Model file for the job. Use its own axes, mm. Coordinates: 2 decimals unless noted, no trailing zeros. Loops run counter-clockwise (first coordinate to the right, second up) from the corner with the lowest first, then second, coordinate; pieces in that order, holes last. Notation, with made-up numbers: (-26.75, 56.5) -> (-0.75, 56.5) arc R21 ccw to (-0.75, 76.5) -> close; hole circle Ø7 at (78.25, 67). An arc over 180 degrees is marked (long way). Use one line per item in the form item = value.
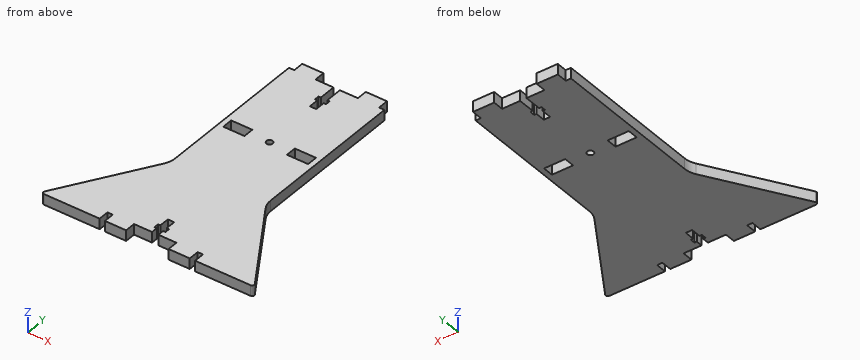
```python
from build123d import *

# Parameters (mm, degrees)
BOSS_EXTRUDE1_DEPTH = 5
SKETCH2_R           = 1.5
SKETCH2_W           = 10
SKETCH2_H           = 5
CUT_EXTRUDE1_DEPTH  = 10
FILLET1_R           = 10
FILLET2_R           = 1


with BuildPart() as part:
    # Sketch1 → Boss-Extrude1 (new body)
    with BuildSketch(Plane.XY):
        Polygon((-32.518889855, -56.191512275), (-30.018889855, -56.191512275), (-30.018889855, -61.191512275), (-20.018889855, -61.191512275), (-20.018889855, -56.191512275), (-11.518889855, -56.191512275), (-11.518889855, -53.191512275), (-12.618889855, -53.191512275), (-12.618889855, -50.891512275), (-11.518889855, -50.891512275), (-11.518889855, -46.191512275), (-8.518889855, -46.191512275), (-8.518889855, -50.891512275), (-7.418889855, -50.891512275), (-7.418889855, -53.191512275), (-8.518889855, -53.191512275), (-8.518889855, -56.191512275), (-0.018889855, -56.191512275), (-0.018889855, -61.191512275), (9.981110145, -61.191512275), (9.981110145, -56.191512275), (12.481110145, -56.191512275), (12.481110145, -61.191512275), (40.481110145, -61.191512275), (12.481110145, -16.103821473), (12.481110145, 58.808487725), (9.981110145, 58.808487725), (9.981110145, 63.808487725), (-0.018889855, 63.808487725), (-0.018889855, 58.808487725), (-8.518889855, 58.808487725), (-8.518889855, 50.808487725), (-7.418889855, 50.808487725), (-7.418889855, 48.508487725), (-8.518889855, 48.508487725), (-8.518889855, 43.808487725), (-11.518889855, 43.808487725), (-11.518889855, 48.508487725), (-12.618889855, 48.508487725), (-12.618889855, 50.808487725), (-11.518889855, 50.808487725), (-11.518889855, 58.808487725), (-20.018889855, 58.808487725), (-20.018889855, 63.808487725), (-30.018889855, 63.808487725), (-30.018889855, 58.808487725), (-32.518889855, 58.808487725), (-32.518889855, -16.103821473), (-60.518889855, -61.191512275), (-32.518889855, -61.191512275), align=None)
    extrude(amount=BOSS_EXTRUDE1_DEPTH)

    # Sketch2 → Cut-Extrude1 (cut)
    with BuildSketch(Plane.XY.offset(5)):
        with Locations((-10.018889855, 16.308487725)):
            Circle(SKETCH2_R)
        with Locations((-25.018889855, 16.308487725)):
            Rectangle(SKETCH2_W, SKETCH2_H)
        with Locations((4.981110145, 16.308487725)):
            Rectangle(SKETCH2_W, SKETCH2_H)
    extrude(amount=-CUT_EXTRUDE1_DEPTH, mode=Mode.SUBTRACT)

    # Fillet1
    fillet1_edges = [part.edges().sort_by_distance(p)[0] for p in [
        (-32.518889855, -16.103821473, 2.5),
        (12.481110145, -16.103821473, 2.5),
    ]]
    fillet(fillet1_edges, radius=FILLET1_R)

    # Fillet2
    fillet2_edges = [part.edges().sort_by_distance(p)[0] for p in [
        (40.481110145, -61.191512275, 2.5),
        (-60.518889855, -61.191512275, 2.5),
    ]]
    fillet(fillet2_edges, radius=FILLET2_R)


solid = part.part
```
Q1. Band-saw the part on D-D, the plane y = 31.5. Write the cut outline in (x, z).
Result:
outline = (-32.52, 0) -> (12.48, 0) -> (12.48, 5) -> (-32.52, 5) -> close
Q2. Band-saw the part on C-C, the plane z = 1.5. State how many separate pieces and enclosed holes the cut face has, and give its area (3 significant figures).
Result:
separate_pieces = 1
enclosed_holes = 3
area = 6,450 mm2
Q3. Pin check, flat tips, straight feed: pin 1 Ø2.5 at (y, z) = (-47.5, 3) entering from -X; pin 2 Ø1.5 at (x, z) = (-6, 1.5) entering from +Y; pin 3 Ø2 at (y, z) = (7.5, 0.5) entering from +X. Stop position of each tip, or through.
Result:
pin_1 = -52.79
pin_2 = 58.81
pin_3 = 12.48
Q4. Wall check: line 1 along X through (y, z) = (18, 2.2); line 2 along X through (y, z) = (48, 4.4); line 3 along Y through (x, z) = (-7.5, 4.8). Give the ranges that are in metal, low to high.
Result:
line_1 = -32.52 to -30.02, -20.02 to -0.02, 9.98 to 12.48
line_2 = -32.52 to -11.52, -8.52 to 12.48
line_3 = -56.19 to -53.19, -50.89 to 48.51, 50.81 to 58.81
Q5. Band-saw the part on B-B, the plane y = 55. Write the cut outline in (x, z), and give its area (3 significant figures).
Result:
outline = (-32.52, 0) -> (-11.52, 0) -> (-11.52, 5) -> (-32.52, 5) -> close; (-8.52, 0) -> (12.48, 0) -> (12.48, 5) -> (-8.52, 5) -> close
area = 210 mm2
Q6. Band-saw the part on A-A, the plane x = -22.5. Write the cut outline in (y, z), and give its area (3 significant figures).
Result:
outline = (-61.19, 0) -> (13.81, 0) -> (13.81, 5) -> (-61.19, 5) -> close; (18.81, 0) -> (63.81, 0) -> (63.81, 5) -> (18.81, 5) -> close
area = 600 mm2
